```python
from build123d import *

# Parameters (mm, degrees)
PER_AGE1_D     = 4
PER_AGE1_DEPTH = 12
PER_AGE1_TIP   = 1.154700538
PER_AGE2_D     = 5.3
PER_AGE2_DEPTH = 1.2
PER_AGE2_TIP   = 1.529978213


with BuildPart() as part:
    # Esquisse1 → Base-Révolution (revolve)
    with BuildSketch(Plane.XY, mode=Mode.PRIVATE) as base_r_volution_sk:
        with BuildLine():
            Line((0.817137041, 3.52228331), (2.6, 4))
            Line((2.6, 4), (28.8, 4))
            Line((28.8, 4), (30, 3.678460969))
            Line((30, 3.678460969), (30, 0))
            Line((30, 0), (0, 0))
            ThreePointArc((0, 0), (0.206961322, 1.807912654), (0.817137041, 3.52228331))
        make_face()
    revolve(base_r_volution_sk.sketch.rotate(Axis((-7.062515413, 0, 0), (1, 0, 0)), 90), axis=Axis((-7.062515413, 0, 0), (1, 0, 0)))

    # Perçage1
    with Locations(Plane(origin=(30, 0, 0), x_dir=(0, 0, -1), z_dir=(1, 0, 0))):
        with Locations((0, 0)):
            Hole(PER_AGE1_D / 2, depth=PER_AGE1_DEPTH)
            with Locations((0, 0, -(PER_AGE1_DEPTH + PER_AGE1_TIP / 2))):  # 120° drill point
                Cone(0, PER_AGE1_D / 2, PER_AGE1_TIP, mode=Mode.SUBTRACT)

    # Perçage2
    with Locations(Plane(origin=(30, 0, 0), x_dir=(0, 0, -1), z_dir=(1, 0, 0))):
        with Locations((0, 0)):
            Hole(PER_AGE2_D / 2, depth=PER_AGE2_DEPTH)
            with Locations((0, 0, -(PER_AGE2_DEPTH + PER_AGE2_TIP / 2))):  # 120° drill point
                Cone(0, PER_AGE2_D / 2, PER_AGE2_TIP, mode=Mode.SUBTRACT)


solid = part.part
```
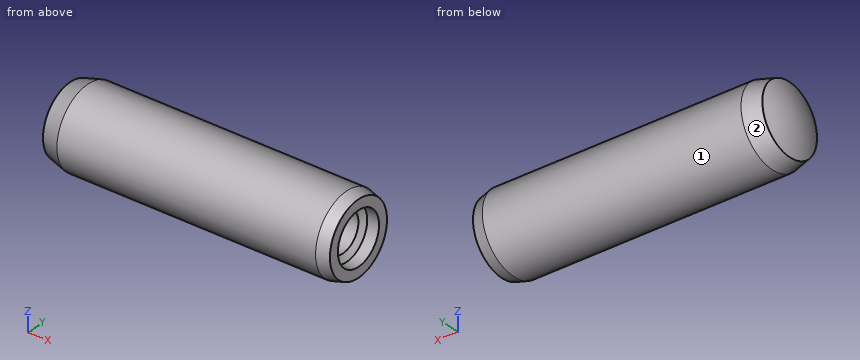
Read the model definition and answer for the solid it produces. Units are mm, in the model's axes. Face numbers are marked on the shaded views. Round coordinates to 2 decimals unless told otherwise and drop trailing zeros. Write each loop counter-clockwise with the first axis right and the second up, starting at its lowest first coordinate (ties: lowest second). Pieces come first, ordered by that corner, then holes. Notation, with made-up numbers: (-15.75, 78.25) -> (40.25, 78.25) arc R25 cw to (40.25, 98.25) -> close; hole circle Ø8 at (66.5, 1). An arc over 180 degrees is marked (long way). Answer in a Markdown table with one row per item. Add a question column.
1) Find section B-B, the plane x = 13.5. Determine the outline of the cut face in (y, z), and give its area (3 significant figures).
2) Determine the mould class of the marked faces 1 and 2 for opening direction X: pulls with the +X half, pulls with the -X half, needs draft (parallel to the pull), parting line crosses it, or undercut.
3) Given P1, Ø1, axis at x = 18, z = 2.5, coming from the +Y side; P2, Ø2, axis at x = 11, z = -0.5, coming from the +Y side; P3, Ø1.5, axis at x = 24, y = -2.5, coming from the +Z side; P4, Ø1.5, axis at y = 0.5, z = -0.5, coming from the +X side, each flat-ended and moving along its own axis, determine where each tip first touches the part or whether it passes through.
4) Consider line 1 (Y direction, x = 25.75, z = 0); line 2 (Y direction, x = 29.4, z = 0); line 3 (Y direction, x = 3.5, z = 2.75). Determine where each line is inside the solid, lowest interval first.
5) Find section A-A, the plane x = 22.5. Determine the outline of the cut face in (y, z), and give its area (3 significant figures).
Findings below:
| question | item | result |
|---|---|---|
| 1 | outline | circle Ø8 at (0, 0) |
| 1 | area | 50.3 mm² |
| 2 | face 1 | needs draft |
| 2 | face 2 | pulls with the -X half |
| 3 | P1 | y = 3.46 |
| 3 | P2 | y = 4 |
| 3 | P3 | z = 3.6 |
| 3 | P4 | x = 17.69 |
| 4 | line 1 | -4 to -2, 2 to 4 |
| 4 | line 2 | -3.84 to -2.65, 2.65 to 3.84 |
| 4 | line 3 | -2.9 to 2.9 |
| 5 | outline | circle Ø8 at (0, 0); hole circle Ø4 at (0, 0) |
| 5 | area | 37.7 mm² |
